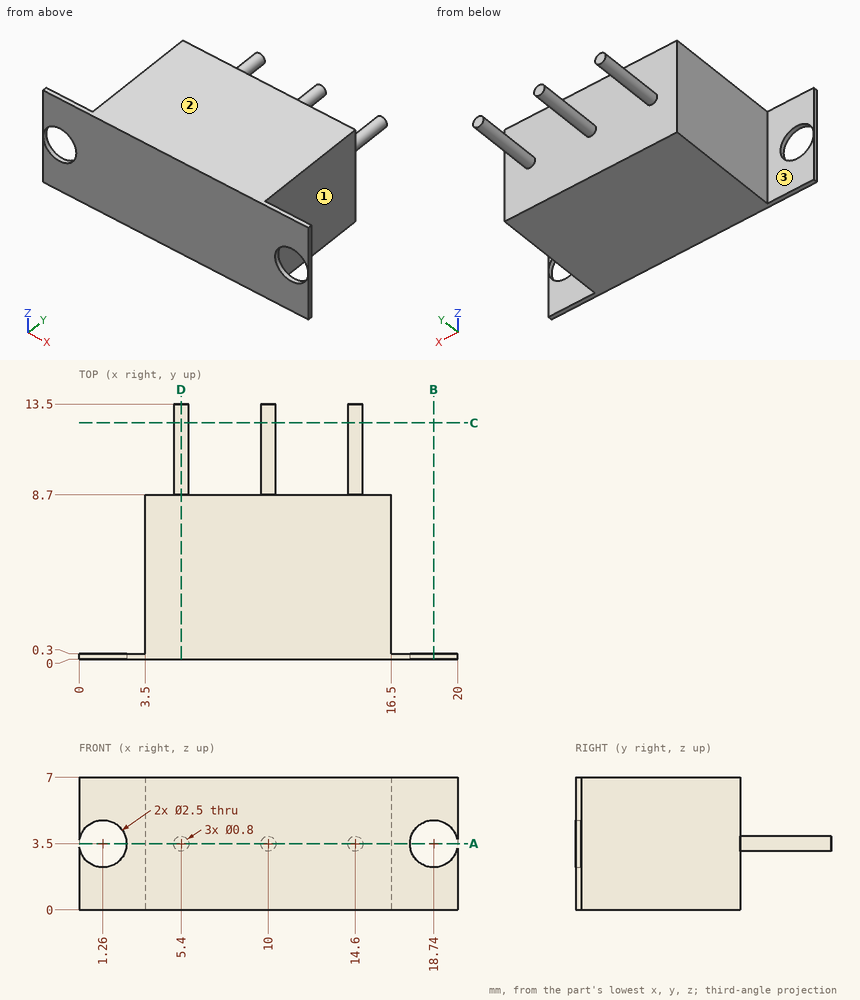
Check sheet for the drawn part. Datum: minimum x, y, z corner. Units: mm. A direction names the side the tool comes from. Round coordinates to 2 decimals unless told otherwise and drop trailing zeros. Order: outer loops, then holes, each group sorted by start corner. A loop starts at its lowest first (then second) coordinate and runs counter-clockwise, first axis right, second up. Notation, with made-up numbers: M 82,71.25 L 90,71.25 A24 cw 90,96.25 Z; hole C -17.75,86 d10. An arc over 180 degrees is marked long. Answer in a Markdown table with one row per item.
(1) Gauge pin test, flat ends, axial feed: pin 1 (3.5 mm diameter, centred on y = 5.5, z = 5, fed in from -X); pin 2 (4 mm diameter, centred on y = 9, z = 3.5, fed in from +X); pin 3 (3 mm diameter, centred on x = 19, z = 2.5, fed in from +Y); pin 4 (5 mm diameter, centred on x = 15.5, y = 9, fed in from +Z). Record the tip position at first contact, or that the pin passes through.
Findings:
| item | result |
|---|---|
| pin 1 | stops at x = 3.5 |
| pin 2 | stops at x = 16.5 |
| pin 3 | stops at y = 0.3 |
| pin 4 | stops at z = 7 |
(2) Section check A-A on z = 3.5. Give the number of separate pieces and of enclosed holes in the cut face, plus the area to 3 significant figures.
Findings:
| item | result |
|---|---|
| separate pieces | 3 |
| enclosed holes | 0 |
| area | 125 mm^2 |
(3) Section check C-C on y = 12.5. Record the boundary of the cut face in (x, z), plus the area to 3 significant figures.
Findings:
| item | result |
|---|---|
| outline | C 5.4,3.5 d0.8; C 10,3.5 d0.8; C 14.6,3.5 d0.8 |
| area | 1.51 mm^2 |
(4) Material ranges on line 1 along Z through (x, y) = (18.74, 0.2); line 2 along Y through (x, z) = (6, 1.75); line 3 along X through (y, z) = (1.25, 6.25), recorded low to high. Write a range as from..to.
Findings:
| item | result |
|---|---|
| line 1 | z = 0..2.25, 4.75..7 |
| line 2 | y = 0..8.7 |
| line 3 | x = 3.5..16.5 |
(5) Section check D-D on x = 5.4. Record the boundary of the cut face in (y, z), plus the area to 3 significant figures.
Findings:
| item | result |
|---|---|
| outline | M 0,0 L 8.7,0 L 8.7,3.1 L 13.5,3.1 L 13.5,3.9 L 8.7,3.9 L 8.7,7 L 0,7 Z |
| area | 64.7 mm^2 |
(6) Set-up check for the marked faces 1, 2 and 3: record each of +Z, -Z, +X, -X, +Y, -Y from which the full face is reachable in a straight line by a thin tool's end or side.
Findings:
| item | result |
|---|---|
| face 1 | +Z, -Z, +X, +Y |
| face 2 | +Z, +X, -X, +Y, -Y |
| face 3 | +Z, -Z, -X, +Y |
(7) Section check B-B on x = 18.74. Record the boundary of the cut face in (y, z), plus the area to 3 significant figures.
Findings:
| item | result |
|---|---|
| outline | M 0,0 L 0.3,0 L 0.3,2.25 L 0,2.25 Z; M 0,4.75 L 0.3,4.75 L 0.3,7 L 0,7 Z |
| area | 1.35 mm^2 |
